For this review, take the finished solid that the model builds, in its own axes (mm). Face numbers are marked on the shaded views. A direction names the side the tool comes from. Give positions to 0.01 mm unless a question says otherwise; leave off trailing zeros. Order: outer loops, then holes, each group sorted by start corner. A loop starts at its lowest first (then second) coordinate and runs counter-clockwise, first axis right, second up.
Item 1: The part is to be moulded in two halves that separate along Z. For the marked faces 4, 5 and 6, say which applies: released by +Z, released by -Z, zero draft, split by the parting line, or undercut.
Item 2: Consider section B-B (x = 0). Give the boundary of the cut face in (y, z), plus the area to 3 significant figures.
Item 3: For probe 1 along Z at (x, y) = (0, 2.25); probe 2 along X at (y, z) = (-5.5, -48); probe 3 along X at (y, z) = (37, -29), list the stretches that pass through material, from the lowest coordinate up.
Item 4: For P1, Ø9.5, axis at x = 0, z = 40.37, coming from the +Y side; P2, Ø10, axis at x = -18.5, y = 18, coming from the +Z side, all flat-tipped, find the tip position at first contact; note any pin that passes through.
Item 5: Consider section C-C (y = 24.5). Give the boundary of the cut face in (x, z), plus the area to 3 significant figures.
Item 6: Consider section D-D (x = 30). Give the boundary of the cut face in (y, z), plus the area to 3 significant figures.
Item 7: Machinability: for the marked faces 1, 2 and 3, which of the approach directions +Z, -Z, +X, -X, +Y, -Y give a long, thin tool a straight path to every point of the face, cutting with its end or side? Answer none if there is none.
Item 8: Consider section A-A (z = -23.5). Give the boundary of the cut face in (x, y).
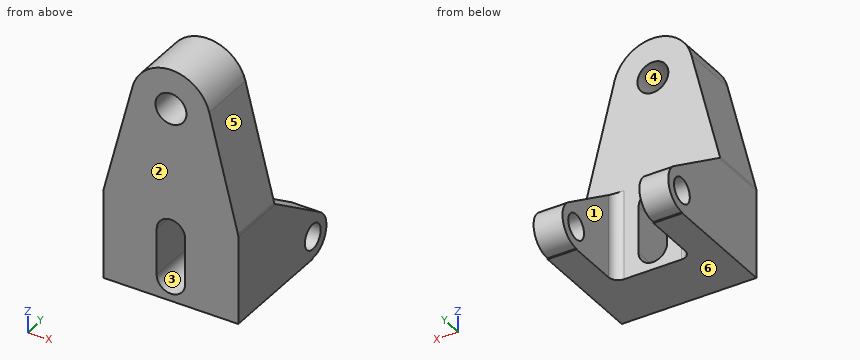
```python
from build123d import *

# Parameters (mm, degrees)
F0_R     = 8.034582
F1_DEPTH = 15
F2_R     = 6.54267
F3_DEPTH = 15
F4_R     = 5.08


with BuildPart() as f1:
    # F0 (on Front) → F1 (new body, symmetric)
    with BuildSketch(Plane.XZ):
        with BuildLine():
            Line((-34.955353, -60.541797), (34.955353, -60.541797))
            Line((34.955353, -60.541797), (34.955353, -14.012067))
            Line((34.955353, -14.012067), (19.885809, 45.410026))
            ThreePointArc((19.885809, 45.410026), (0, 60.882263), (-19.885809, 45.410026))
            Line((-19.885809, 45.410026), (-34.955353, -14.012067))
            Line((-34.955353, -14.012067), (-34.955353, -60.541797))
        make_face()
        with BuildLine():
            ThreePointArc((-7.400118, -25.208272), (0, -17.808154), (7.400118, -25.208272))
            Line((7.400118, -25.208272), (7.400118, -49.345592))
            ThreePointArc((7.400118, -49.345592), (0, -56.74571), (-7.400118, -49.345592))
            Line((-7.400118, -49.345592), (-7.400118, -25.208272))
        make_face(mode=Mode.SUBTRACT)
        with Locations((0, 40.366952)):
            Circle(F0_R, mode=Mode.SUBTRACT)
    extrude(amount=F1_DEPTH, both=True)

    # F2 (on face) → F3 (join)
    with BuildSketch(Plane.YZ.offset(34.955353)):
        with BuildLine():
            Line((53.032903, -39.416735), (15, -14.012067))
            Line((15, -14.012067), (15, -60.541797))
            Line((15, -60.541797), (46.407126, -60.541797))
            Line((46.407126, -60.541797), (46.545673, -60.100067))
            ThreePointArc((46.545673, -60.100067), (57.536015, -52.188126), (53.032903, -39.416735))
        make_face()
        with Locations((46.759732, -48.808195)):
            Circle(F2_R, mode=Mode.SUBTRACT)
    extrude(amount=-F3_DEPTH)

    # F4
    f4_edges = [f1.edges().sort_by_distance(p)[0] for p in [
        (19.955353, 15, -37.276932),
        (-34.955353, 0, -14.012067),
        (34.955353, 0, -14.012067),
    ]]
    fillet(f4_edges, radius=F4_R)

    # F5: F1 across plane


with BuildPart() as f1_1:
    add(f1.part)
    add(f1.part.mirror(Plane.YZ))


solid = f1_1.part
```
Resolved:
1. face 4: undercut
1. face 5: released by +Z
1. face 6: released by -Z
2. outline: (-15, -60.54) - (15, -60.54) - (15, -56.75) - (-15, -56.75) - close; (-15, -17.81) - (15, -17.81) - (15, 32.33) - (-15, 32.33) - close; (-15, 48.4) - (15, 48.4) - (15, 60.88) - (-15, 60.88) - close
2. area: 1,990 mm2
3. probe 1: z = -60.54 to -56.75, -17.81 to 32.33, 48.4 to 60.88
3. probe 2: x = -34.96 to -7.4, 7.4 to 34.96
3. probe 3: x = -34.96 to -19.96, 19.96 to 34.96
4. P1: passes through
4. P2: stops at z = 54.88
5. outline: (-34.96, -60.54) - (-19.96, -60.54) - (-19.96, -20.36) - (-34.96, -20.36) - close; (19.96, -60.54) - (34.96, -60.54) - (34.96, -20.36) - (19.96, -20.36) - close
5. area: 1,210 mm2
6. outline: (-15, -60.54) - (46.41, -60.54) - (46.55, -60.1) arc R11.29 ccw to (53.03, -39.42) - (15, -14.01) - (15, 5.53) - (-15, 5.53) - close; hole circle Ø13.09 at (46.76, -48.81)
6. area: 3,190 mm2
7. face 1: +Z, -Z, +Y
7. face 2: +Z, -Z, +X, -X, -Y
7. face 3: +Y, -Y
8. outline: (-34.96, -15) - (-7.2, -15) - (-7.2, 15) - (-14.88, 15) arc R5.08 cw to (-19.96, 20.08) - (-19.96, 29.2) - (-34.96, 29.2) - close; (7.2, -15) - (34.96, -15) - (34.96, 29.2) - (19.96, 29.2) - (19.96, 20.08) arc R5.08 cw to (14.88, 15) - (7.2, 15) - close
